from build123d import *

# Parameters (mm, degrees)
F0_R     = 42.1551609163
F0_R_2   = 36.6737913898
F1_DEPTH = 101.6
F2_R     = 36.6906853339
F3_DEPTH = 0.254


# Not quite as in the source:
# - the program builds the solid bodies; features that only make, move or delete a surface that nothing else refers to are left out


with BuildPart() as f1:
    # F0 (on Front) → F1 (new body)
    with BuildSketch(Plane.XZ):
        Circle(F0_R)
        Circle(F0_R_2, mode=Mode.SUBTRACT)
    extrude(amount=-F1_DEPTH)

    # F2 (on face) → F3 (join)
    with BuildSketch(Plane(origin=(0, 101.6, 0), x_dir=(-1, 0, 0), z_dir=(0, 1, 0))):
        Circle(F2_R)
    extrude(amount=F3_DEPTH)


solid = f1.part
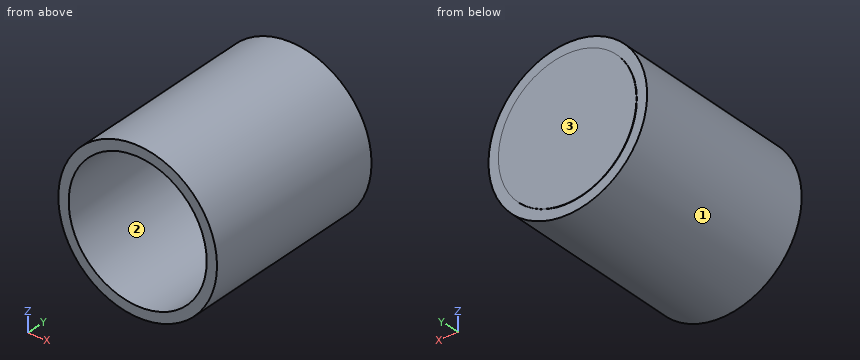
Work out the finished part from the listing and answer in its coordinate system (mm). Face numbers are marked on the shaded views. Round coordinates to 2 decimals unless told otherwise and drop trailing zeros. Write each loop counter-clockwise with the first axis right and the second up, starting at its lowest first coordinate (ties: lowest second). Pieces come first, ordered by that corner, then holes. Notation, with made-up numbers: (27, 15.5) -> (67, 15.5) arc R13 ccw to (67, 28.5) -> close; hole circle Ø1 at (-10.75, 6). An arc over 180 degrees is marked (long way). Answer as CSV lines item,"result". Start each with the question number.
(1) Each of these flat-tipped pins is pushed along its axis until it touches: pin 1 (3 mm diameter, centred on x = -6.5, y = 86.5, fed in from +Z); pin 2 (10 mm diameter, centred on x = 13.5, z = 24, fed in from -Y); pin 3 (2 mm diameter, centred on x = 21, y = 10.5, fed in from +Z). Where does it stop, or does it pass through?
(2) Find the intervals of material crossed by probe 1 along Z at (x, y) = (0, 43.5); probe 2 along Z at (x, y) = (-1, 76); probe 3 along Y at (x, z) = (14.5, -25.5), in increasing order.
(3) The part is cut by section B-B, the plane y = 87. Give the vertices of the cut face in (x, z), then the cut area to 3 significant figures.
(4) The part is cut by section A-A, the plane x = 0. Give the vertices of the cut face in (y, z).
(5) The part is cut by section C-C, the plane z = 0. Give the vertices of the cut face in (x, y).
(6) The mould has two halves that part along Z. Classify the marked faces 1, 2 and 3: +Z half, -Z half, draft (parallel to the pull), parting line (faces both ways), or undercut.
Output values:
1,pin 1,"stops at z = 41.86"
1,pin 2,"stops at y = 101.6"
1,pin 3,"stops at z = 37.11"
2,probe 1,"z = -42.16 to -36.67, 36.67 to 42.16"
2,probe 2,"z = -42.14 to -36.66, 36.66 to 42.14"
2,probe 3,"y = 101.6 to 101.85"
3,outline,"circle Ø84.31 at (0, 0); hole circle Ø73.35 at (0, 0)"
3,area,"1,360 mm²"
4,outline,"(0, -42.16) -> (101.6, -42.16) -> (101.6, -36.69) -> (101.85, -36.69) -> (101.85, 36.69) -> (101.6, 36.69) -> (101.6, 42.16) -> (0, 42.16) -> (0, 36.67) -> (101.6, 36.67) -> (101.6, -36.67) -> (0, -36.67) -> close"
5,outline,"(-42.16, 0) -> (-36.67, 0) -> (-36.67, 101.6) -> (36.67, 101.6) -> (36.67, 0) -> (42.16, 0) -> (42.16, 101.6) -> (36.69, 101.6) -> (36.69, 101.85) -> (-36.69, 101.85) -> (-36.69, 101.6) -> (-42.16, 101.6) -> close"
6,face 1,"parting line"
6,face 2,"undercut"
6,face 3,"draft"
